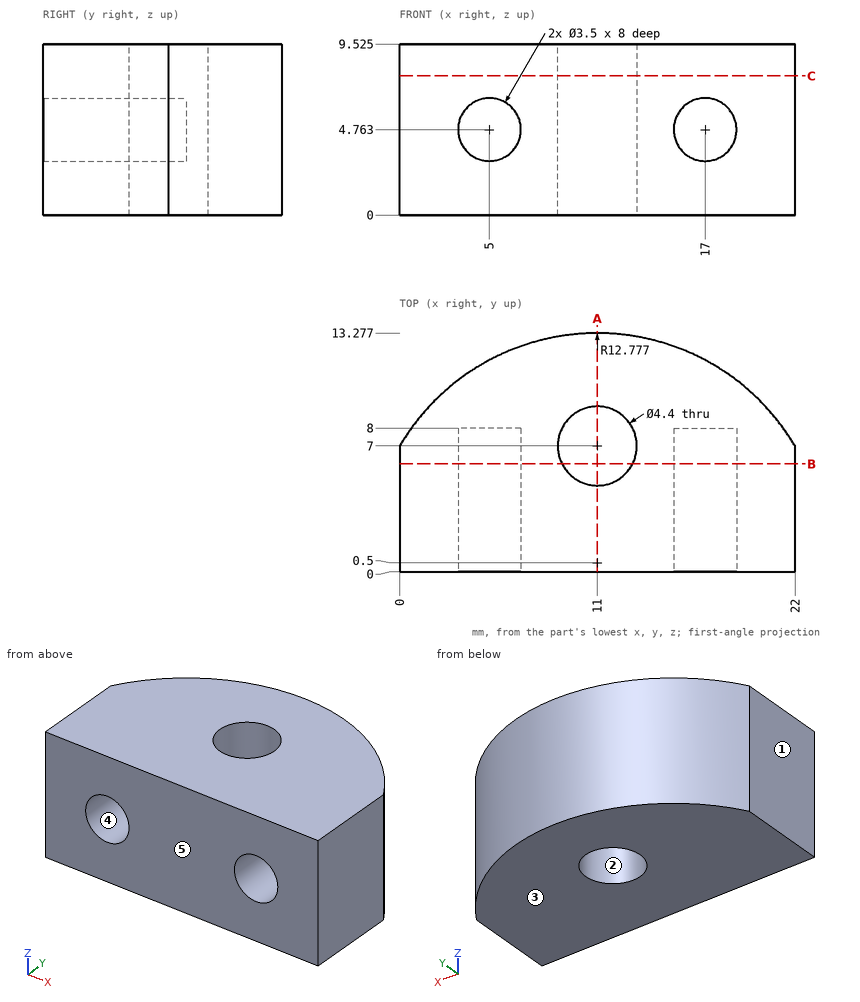
For this review, use the dimensioned drawing (mm, ordinates from the lowest corner) and the shaded views. A direction names the side the tool comes from. Coordinates: 2 decimals unless noted, no trailing zeros. Write each loop counter-clockwise with the first axis right and the second up, starting at its lowest first coordinate (ties: lowest second). Pieces come first, ordered by that corner, then holes. Notation, with made-up numbers: (4.5, -22) - (8.5, -22) arc R14 ccw to (8.5, -14) - close; hole circle Ø2 at (-37.5, 54). An arc over 180 degrees is marked (long way). Answer in a Markdown table with one row per item. Add a question column.
Q1. For the marked faces 4 and 5, list the 3-axis set-ups (+Z, -Z, +X, -X, +Y, -Y) from which the entire face can be reached by the end or side of a thin tool; tool diameter is ignored.
Q2. Clearance check with flat-ended pins moving along their axes: pin 1 (1 mm diameter, centred on x = 16.5, z = 5.5, fed in from -Y); pin 2 (2 mm diameter, centred on x = 4, z = 8.5, fed in from +Y); pin 3 (1 mm diameter, centred on x = 17, z = 1.5, fed in from +Y). State where each tip first meets the part, or that it passes through.
Q3. Consider section B-B on y = 6. Give the number of separate pieces and of enclosed holes in the cut face, then the cut area to 3 significant figures.
Q4. Draft analysis for pull direction X (two halves, no side actions). For the marked faces 1, 2 and 3, state which applies: +X half, -X half, draft (parallel to the pull), parting line (faces both ways), or undercut.
Q5. Consider section A-A on x = 11. Give the boundary of the cut face in (y, z) (1 decimal).
Q6. To check wall thickness, follow line 1 along Z through (x, y) = (17, 4.5) (1 decimal); line 2 along Y through (x, z) = (11, 3.5); line 3 along X through (y, z) = (5.5, 5.5) (1 decimal). State the ranges of each line that lie inside material, in increasing order. Write a range as from..to.
Q7. Consider section C-C on z = 7.75. Give the boundary of the cut face in (x, y), then the cut area to 3 significant figures.
Answers below:
| question | item | result |
|---|---|---|
| 1 | face 4 | -Y |
| 1 | face 5 | +Z, -Z, +X, -X, -Y |
| 2 | pin 1 | y = 8 |
| 2 | pin 2 | y = 11.78 |
| 2 | pin 3 | y = 12.03 |
| 3 | separate pieces | 2 |
| 3 | enclosed holes | 2 |
| 3 | area | 153 mm² |
| 4 | face 1 | -X half |
| 4 | face 2 | undercut |
| 4 | face 3 | draft |
| 5 | outline | (0, 0) - (4.8, 0) - (4.8, 9.5) - (0, 9.5) - close; (9.2, 0) - (13.3, 0) - (13.3, 9.5) - (9.2, 9.5) - close |
| 6 | line 1 | 0..3, 6.5..9.5 |
| 6 | line 2 | 0..4.8, 9.2..13.28 |
| 6 | line 3 | 0..3.4, 6.6..9.4, 12.6..15.4, 18.6..22 |
| 7 | outline | (0, 0) - (22, 0) - (22, 7) arc R12.78 ccw to (0, 7) - close; hole circle Ø4.4 at (11, 7) |
| 7 | area | 237 mm² |
